Geometry check sheet. Reference: the model listing, model coordinates, mm. Give positions to 0.01 mm unless a question says otherwise; leave off trailing zeros. Loops run counter-clockwise (first coordinate to the right, second up) from the corner with the lowest first, then second, coordinate; pieces in that order, holes last.
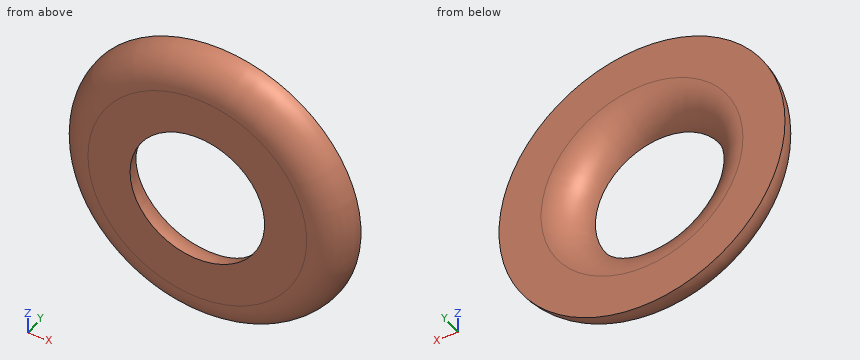
Autodesk Inventor part; units mm, degrees
ref_plane "YZ Plane" through (0, 0, 0) normal (1, 0, 0) x (0, 1, 0)
ref_plane "XZ Plane" through (0, 0, 0) normal (0, 1, 0) x (-1, 0, 0)
ref_plane "XY Plane" through (0, 0, 0) normal (0, 0, 1) x (1, 0, 0)
sketch "Boceto1" plane through (0, 0, 0) normal (0, 1, 0) x (-1, 0, 0)
  circle A0 centre (0, 0) radius 4
  circle A1 centre (0, 0) radius 8.5
  dimension "d0" = 8
  dimension "d1" = 17
extrude "Extrusión1" add sketch "Boceto1" along normal blind 2
fillet "Empalme1" radius 2 1 edges at (8.5, 0, 0)
fillet "Empalme2" radius 2 1 edges at (4, 2, 0)
properties part number "BASE_ARANDELA"
1) Sectioned sample at C-C on y = 1.65. Enter the section's corners in (x, z).
2) Sectioned sample at D-D on y = 0.5. Enter the section's corners in (x, z), plus the area to 3 significant figures.
3) Depth check by flat-ended pin: P1, Ø5, axis at x = 2, z = 0.5, coming from the +Y side; P2, Ø2, axis at x = 6, z = -5.5, coming from the -Y side. Enter the tip coordinate at first touch or a pass-through.
4) Scan lines: line 1 along Z through (x, y) = (3.5, 0.65); line 2 along X through (y, z) = (1.2, 0.75); line 3 along X through (y, z) = (1.45, -1). Record each from-to range of solid material in increasing order.
Determined:
1. outline: circle Ø16.94 at (0, 0); hole circle Ø9.74 at (0, 0)
2. outline: circle Ø15.65 at (0, 0); hole circle Ø8.13 at (0, 0)
2. area: 140 mm2
3. P1: stops at y = 1.39
3. P2: stops at y = 0.1
4. line 1: z = -7.17 to -2.15, 2.15 to 7.17
4. line 2: x = -8.3 to -4.34, 4.34 to 8.3
4. line 3: x = -8.36 to -4.51, 4.51 to 8.36
